```python
from build123d import *

# Parameters (mm, degrees)
SKETCH1_W                      = 20
SKETCH1_H                      = 28.4
BACK_WALL_DEPTH                = 3.8
SKETCH3_W                      = 20
SKETCH3_H                      = 4
BOTTOM_WALL_DEPTH              = 24.5
LEFT_WALL_DEPTH                = 2.5
SKETCH6_W                      = 6.5
SKETCH6_H                      = 9.5
BOTTOM_CONNECTION_CUTOUT_DEPTH = 11
SKETCH7_W                      = 7
SKETCH7_H                      = 9.9
TOP_CONNECTION_CUTOUT_DEPTH    = 11
SKETCH8_W                      = 6
SKETCH8_H                      = 2
BOTTOM_NOTCH_DEPTH             = 3
SKETCH9_W                      = 6
SKETCH9_H                      = 2
TOP_NOTCH_DEPTH                = 3
FILLET1_R                      = 1
BOTTOM_LIGHTENING_CUTOUT_DEPTH = 3
CUT_EXTRUDE2_DEPTH             = 2


with BuildPart() as part:
    # Sketch1 → back_wall (new body)
    with BuildSketch(Plane.XY):
        Rectangle(SKETCH1_W, SKETCH1_H)
    extrude(amount=BACK_WALL_DEPTH)

    # Sketch3 → bottom_wall (add)
    with BuildSketch(Plane.XY.offset(3.8)):
        with Locations((0, -12.2)):
            Rectangle(SKETCH3_W, SKETCH3_H)
    extrude(amount=BOTTOM_WALL_DEPTH)

    # Sketch4 → left_wall (add)
    with BuildSketch(Plane.ZY.offset(10)):
        Polygon((3.8, 14.2), (7.2, 14.2), (28.3, -7.2), (28.3, -10.2), (3.8, -10.2), align=None)
    left_wall = extrude(amount=-LEFT_WALL_DEPTH)

    # right_wall: left_wall across plane
    add(left_wall.mirror(Plane(origin=(0, 0, 0), x_dir=(0, 0, 1), z_dir=(1, 0, 0))))

    # Sketch6 → bottom_connection_cutout (cut)
    with BuildSketch(Plane(origin=(0, -10.2, 0), x_dir=(1, 0, 0), z_dir=(0, 1, 0))):
        with Locations((0, -14.75)):
            Rectangle(SKETCH6_W, SKETCH6_H)
    extrude(amount=-BOTTOM_CONNECTION_CUTOUT_DEPTH, mode=Mode.SUBTRACT)

    # Sketch7 → top_connection_cutout (cut)
    with BuildSketch(Plane.XY.offset(3.8)):
        with Locations((0, 0.75)):
            Rectangle(SKETCH7_W, SKETCH7_H)
    extrude(amount=-TOP_CONNECTION_CUTOUT_DEPTH, mode=Mode.SUBTRACT)

    # Sketch8 → bottom_notch (add)
    with BuildSketch(Plane.XZ.offset(14.2)):
        with Locations((0, 25.3)):
            Rectangle(SKETCH8_W, SKETCH8_H)
        with Locations((0, 3.3)):
            Rectangle(SKETCH8_W, SKETCH8_H)
    extrude(amount=BOTTOM_NOTCH_DEPTH)

    # Sketch9 → top_notch (add)
    with BuildSketch(Plane(origin=(0, 0, 0), x_dir=(-1, 0, 0), z_dir=(0, 0, -1))):
        with Locations((0, -11.2)):
            Rectangle(SKETCH9_W, SKETCH9_H)
        with Locations((0, 10.8)):
            Rectangle(SKETCH9_W, SKETCH9_H)
    extrude(amount=TOP_NOTCH_DEPTH)

    # Fillet1
    fillet1_edges = [part.edges().sort_by_distance(p)[0] for p in [
        (3, 9.8, -1.5),
        (3, 11.8, -1.5),
        (-3, 11.8, -1.5),
        (-3, 9.8, -1.5),
        (-3, -12.2, -1.5),
        (-3, -10.2, -1.5),
        (3, -10.2, -1.5),
        (3, -12.2, -1.5),
        (3, -15.7, 4.3),
        (3, -15.7, 2.3),
        (-3, -15.7, 4.3),
        (-3, -15.7, 2.3),
        (-3, -15.7, 26.3),
        (-3, -15.7, 24.3),
        (3, -15.7, 26.3),
        (3, -15.7, 24.3),
    ]]
    fillet(fillet1_edges, radius=FILLET1_R - 0.0001)  # a hair under: the kernel refuses the full size

    # Sketch11 → bottom_lightening_cutout (cut)
    with BuildSketch(Plane.XZ.offset(14.2)):
        with BuildLine():
            Line((2, 2.3), (6, 2.3))
            Line((6, 2.3), (6, 8.3))
            Line((6, 8.3), (-6, 8.3))
            Line((-6, 8.3), (-6, 2.3))
            Line((-6, 2.3), (-2, 2.3))
            ThreePointArc((-2, 2.3), (-2.707106781, 2.592893219), (-3, 3.3))
            ThreePointArc((-3, 3.3), (-2.707106781, 4.007106781), (-2, 4.3))
            Line((-2, 4.3), (2, 4.3))
            ThreePointArc((2, 4.3), (2.707106781, 4.007106781), (3, 3.3))
            ThreePointArc((3, 3.3), (2.707106781, 2.592893219), (2, 2.3))
        make_face()
        with BuildLine():
            Line((-6, 20.3), (6, 20.3))
            Line((6, 20.3), (6, 26.3))
            Line((6, 26.3), (2, 26.3))
            ThreePointArc((2, 26.3), (2.707106781, 26.007106781), (3, 25.3))
            ThreePointArc((3, 25.3), (2.707106781, 24.592893219), (2, 24.3))
            Line((2, 24.3), (-2, 24.3))
            ThreePointArc((-2, 24.3), (-2.707106781, 24.592893219), (-3, 25.3))
            ThreePointArc((-3, 25.3), (-2.707106781, 26.007106781), (-2, 26.3))
            Line((-2, 26.3), (-6, 26.3))
            Line((-6, 26.3), (-6, 20.3))
        make_face()
    extrude(amount=-BOTTOM_LIGHTENING_CUTOUT_DEPTH, mode=Mode.SUBTRACT)

    # Sketch13 → Cut-Extrude2 (cut)
    with BuildSketch(Plane(origin=(0, 0, 0), x_dir=(-1, 0, 0), z_dir=(0, 0, -1))):
        with BuildLine():
            Line((-2, 11.8), (-6, 11.8))
            Line((-6, 11.8), (-6, 7.8))
            Line((-6, 7.8), (6, 7.8))
            Line((6, 7.8), (6, 11.8))
            Line((6, 11.8), (2, 11.8))
            ThreePointArc((2, 11.8), (2.707106781, 11.507106781), (3, 10.8))
            ThreePointArc((3, 10.8), (2.707106781, 10.092893219), (2, 9.8))
            Line((2, 9.8), (-2, 9.8))
            ThreePointArc((-2, 9.8), (-2.707106781, 10.092893219), (-3, 10.8))
            ThreePointArc((-3, 10.8), (-2.707106781, 11.507106781), (-2, 11.8))
        make_face()
        with BuildLine():
            Line((6, -6.2), (-6, -6.2))
            Line((-6, -6.2), (-6, -12.2))
            Line((-6, -12.2), (-2, -12.2))
            ThreePointArc((-2, -12.2), (-2.707106781, -11.907106781), (-3, -11.2))
            ThreePointArc((-3, -11.2), (-2.707106781, -10.492893219), (-2, -10.2))
            Line((-2, -10.2), (2, -10.2))
            ThreePointArc((2, -10.2), (2.707106781, -10.492893219), (3, -11.2))
            ThreePointArc((3, -11.2), (2.707106781, -11.907106781), (2, -12.2))
            Line((2, -12.2), (6, -12.2))
            Line((6, -12.2), (6, -6.2))
        make_face()
    extrude(amount=-CUT_EXTRUDE2_DEPTH, mode=Mode.SUBTRACT)


solid = part.part
```
Could you check a few things on this model? Use its own coordinates, in mm. A direction names the side the tool comes from. Give positions to 0.01 mm unless a question says otherwise; leave off trailing zeros. Order: outer loops, then holes, each group sorted by start corner. A loop starts at its lowest first (then second) coordinate and runs counter-clockwise, first axis right, second up.
Q1. Suppose I cut it at D-D, the plane y = 2. Write out the boundary of the cut face in (x, z), and give its area (3 significant figures).
Q2. Suppose I cut it at A-A, the plane y = -13. Write out the boundary of the cut face in (x, z), and give its area (3 significant figures).
Q3. I'm going to push flat-ended pins straight in: P1, Ø3, axis at x = -4.5, y = 8.5, coming from the +Z side; P2, Ø0.9, axis at x = 0.5, z = -1.5, coming from the -Y side; P3, Ø1.1, axis at x = 2.5, z = 26, coming from the +Y side; P4, Ø1, axis at y = 5, z = 16.5, coming from the +X side. Where does each tip first touch, or does it pass through?
Q4. Suppose I cut it at C-C, the plane x = -1.5. Count the separate pieces of the cut face and the enclosed holes in it, and give its area (3 significant figures).
Q5. We'd pull the mould along X, two halves only. Please class faces 6 (the flat face through (-8.77, 3.65, 17.6)), 7 (the cylindrical face through (-2.699, 11.515, -1.521)), 8 (the flat face through (-6, -13, 5)): +X half, -X half, draft (parallel to the pull), parting line (faces both ways), or undercut.
Q6. If I drill on line 1 along Z through (x, y) = (4.5, -13); line 2 along X through (y, z) = (13, 6); line 3 along Z through (x, y) = (0.25, -10.5), over which ranges is the centre line in solid material (lowest first)?
Q7. For faces 1 (the flat face through (6, 10, 1)), 2 (the flat face through (-7.5, -1, 13)), 3 (the flat face through (8.77, 3.65, 17.6)), 4 (the flat face through (0, -12, 19.5)), 5 (the flat face through (0, -14, 24.3)), which set-ups out of +Z, -Z, +X, -X, +Y, -Y let a thin tool reach every point of the face, with its end or its side?
Solution:
1. outline: (-10, 0) - (-3.5, 0) - (-3.5, 3.8) - (-7.5, 3.8) - (-7.5, 19.23) - (-10, 19.23) - close; (3.5, 0) - (10, 0) - (10, 19.23) - (7.5, 19.23) - (7.5, 3.8) - (3.5, 3.8) - close
1. area: 127 mm2
2. outline: (-10, 0) - (10, 0) - (10, 28.3) - (-10, 28.3) - close; hole (-6, 2.3) - (-2, 2.3) arc R1 cw to (-2, 4.3) - (2, 4.3) arc R1 cw to (2, 2.3) - (6, 2.3) - (6, 8.3) - (-6, 8.3) - close; hole (-6, 20.3) - (6, 20.3) - (6, 26.3) - (2, 26.3) arc R1 cw to (2, 24.3) - (-2, 24.3) arc R1 cw to (-2, 26.3) - (-6, 26.3) - close; hole (-3.25, 10) - (3.25, 10) - (3.25, 19.5) - (-3.25, 19.5) - close
2. area: 383 mm2
3. P1: stops at z = 3.8
3. P2: stops at y = -12.2
3. P3: stops at y = -10.2
3. P4: stops at x = 10
4. separate pieces: 3
4. enclosed holes: 0
4. area: 118 mm2
5. face 6: draft
5. face 7: -X half
5. face 8: undercut
6. line 1: z = 0 to 2.3, 8.3 to 20.3, 26.3 to 28.3
6. line 2: x = -10 to -7.5, 7.5 to 10
6. line 3: z = -3 to 10, 19.5 to 28.3
7. face 1: -Z
7. face 2: +Z, +Y
7. face 3: +Z, +X, -X, +Y
7. face 4: +Y, -Y
7. face 5: -Y
